from build123d import *

# Parameters (mm, degrees)
SALIENTE_EXTRUIR1_DEPTH    = 1.75
CROQUIS2_W                 = 17.5
CROQUIS2_H                 = 15.2
CROQUIS2_W_2               = 9.5
CROQUIS2_H_2               = 22
CROQUIS2_W_3               = 40
CROQUIS2_H_3               = 5
CROQUIS2_W_4               = 25
CORTAR_EXTRUIR1_DEPTH      = 0.2
CORTAR_EXTRUIR2_DEPTH      = 168.824208623
CORTAR_EXTRUIR2_DEPTH_BACK = 168.824208623
CROQUIS3_R                 = 2.2


with BuildPart() as part:
    # Croquis1 → Saliente-Extruir1 (new body)
    with BuildSketch(Plane.XY):
        Polygon((0, 0), (75.25, 0), (75.25, 150), (1.65, 150), align=None)
    extrude(amount=SALIENTE_EXTRUIR1_DEPTH)

    # Croquis2 → Cortar-Extruir1 (cut)
    with BuildSketch(Plane.XY.offset(1.75)):
        with Locations((66.5, 7.6)):
            Rectangle(CROQUIS2_W, CROQUIS2_H)
        with Locations((4.75, 11)):
            Rectangle(CROQUIS2_W_2, CROQUIS2_H_2)
        with Locations((21.65, 147.5)):
            Rectangle(CROQUIS2_W_3, CROQUIS2_H_3)
        with Locations((62.75, 147.5)):
            Rectangle(CROQUIS2_W_4, CROQUIS2_H_3)
    extrude(amount=-CORTAR_EXTRUIR1_DEPTH, mode=Mode.SUBTRACT)

    # Croquis3 → Cortar-Extruir2 (cut, two sides: drawn at the far end of the back side and taken through both)
    with BuildSketch(Plane.XY.offset(1.55).offset(-CORTAR_EXTRUIR2_DEPTH_BACK)):
        with Locations((3.650817793, 4.6)):
            Circle(CROQUIS3_R)
        with Locations((70.45, 5.8)):
            Circle(CROQUIS3_R)
        with Locations((5.35, 145.2)):
            Circle(CROQUIS3_R)
        with Locations((70.55, 145.8)):
            Circle(CROQUIS3_R)
    extrude(amount=CORTAR_EXTRUIR2_DEPTH + CORTAR_EXTRUIR2_DEPTH_BACK, mode=Mode.SUBTRACT)


solid = part.part
Geometry check sheet. Reference: the model listing, model coordinates, mm. A direction names the side the tool comes from. Give positions to 0.01 mm unless a question says otherwise; leave off trailing zeros. Write each loop counter-clockwise with the first axis right and the second up, starting at its lowest first coordinate (ties: lowest second). Pieces come first, ordered by that corner, then holes.
1) Thickness scan on line 1 (X direction, y = 4.6, z = 0.8); line 2 (Y direction, x = 72, z = 1.2); line 3 (X direction, y = 5.8, z = 1.2). Record the ranges inside material, lowest first.
Values follow:
line 1: x = 0.05 to 1.45, 5.85 to 68.61, 72.29 to 75.25
line 2: y = 0 to 4.24, 7.36 to 144.15, 147.45 to 150
line 3: x = 0.06 to 1.81, 5.49 to 68.25, 72.65 to 75.25
2) Release check for a two-part mould opening along X. For faces 1 (the face through (1.453, 4.697, 0.764)), 2 (the face through (63, 148, 1.55)), 3 (the face through (68.252, 5.897, 0.764)) record: released by +X, released by -X, zero draft, split by the parting line, or undercut.
Values follow:
face 1: undercut
face 2: zero draft
face 3: undercut
3) Cross-section at C-C (y = 105). Record the boundary of the cut face in (x, z) (3 decimals).
Values follow:
outline: (1.155, 0) - (75.25, 0) - (75.25, 1.75) - (1.155, 1.75) - close
4) Cross-section at B-B (x = 70.55). Record the boundary of the cut face in (y, z).
Values follow:
outline: (0, 0) - (3.6, 0) - (3.6, 1.55) - (0, 1.55) - close; (8, 0) - (143.6, 0) - (143.6, 1.75) - (15.2, 1.75) - (15.2, 1.55) - (8, 1.55) - close; (148, 0) - (150, 0) - (150, 1.55) - (148, 1.55) - close
5) Cross-section at A-A (z = 1). Record the boundary of the cut face in (x, y), plus the area to 3 significant figures.
Values follow:
outline: (0, 0) - (75.25, 0) - (75.25, 150) - (1.65, 150) - close; hole circle Ø4.4 at (3.65, 4.6); hole circle Ø4.4 at (5.35, 145.2); hole circle Ø4.4 at (70.45, 5.8); hole circle Ø4.4 at (70.55, 145.8)
area: 11,100 mm2
6) Set-up check for faces 4 (the face through (21, 148, 1.55)), 5 (the face through (5, 11, 1.55)), 6 (the face through (66, 8, 1.55)), 7 (the face through (6.37, 143.25, 0.86)): record each of +Z, -Z, +X, -X, +Y, -Y from which the full face is reachable in a straight line by a thin tool's end or side.
Values follow:
face 4: +Z, +Y
face 5: +Z, -X, -Y
face 6: +Z, +X, -Y
face 7: +Z, -Z
7) Go/stop test with a flat-tipped pin: pin 1 Ø16.5 at (x, y) = (68.5, 5) entering from +Z. Record where the tip stops, or that it passes through.
Values follow:
pin 1: stops at z = 1.55
